Verification items for the finished model (mm, model axes). Face numbers are marked on the shaded views. A direction names the side the tool comes from. Give positions to 0.01 mm unless a question says otherwise; leave off trailing zeros. Loops run counter-clockwise (first coordinate to the right, second up) from the corner with the lowest first, then second, coordinate; pieces in that order, holes last. Notation, with made-up numbers: (50.5, 82.5) -> (69.5, 82.5) arc R17 ccw to (69.5, 110.5) -> close; hole circle Ø11 at (5.5, -5). An arc over 180 degrees is marked (long way). Answer in a Markdown table with one row per item. Add a question column.
Q1. Section check C-C on z = 15.75. Enter the section's corners in (x, y).
Q2. Gauge pin test, flat ends, axial feed: P1, Ø2, axis at x = 29, y = 16, coming from the +Z side; P2, Ø6, axis at y = -17.5, z = 4, coming from the -X side. Record the tip position at first contact, or that the pin passes through.
Q3. Section check A-A on y = -22.5. Enter the section's corners in (x, z), and give its area (3 significant figures).
Q4. Section check D-D on y = -3. Enter the section's corners in (x, z), and give its area (3 significant figures).
Q5. Set-up check for the marked faces 1, 2 and 3: record each of +Z, -Z, +X, -X, +Y, -Y from which the full face is reachable in a straight line by a thin tool's end or side.
Q6. Material ranges on probe 1 along Y at (x, z) = (-17, 12.5); probe 2 along X at (y, z) = (19, 14.5); probe 3 along Y at (x, z) = (-24, 7.75), recorded low to high.
Q7. Release check for a two-part mould opening along X. For the marked faces 4, 5 and 6 record: pulls with the +X half, pulls with the -X half, needs draft (parallel to the pull), parting line crosses it, or undercut.
Q8. Section check B-B on x = 12. Enter the section's corners in (y, z), and give its area (3 significant figures).
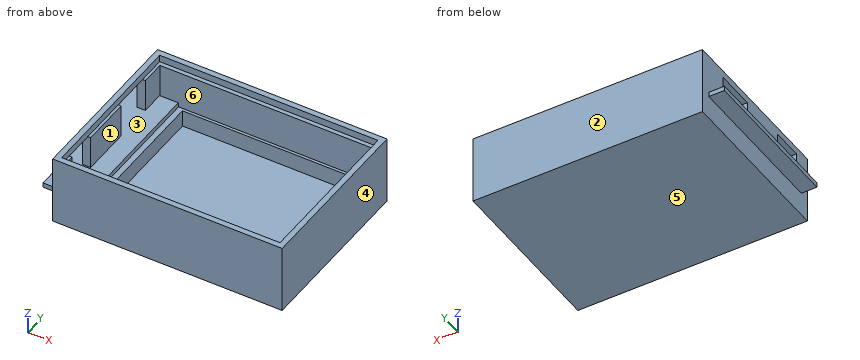
```python
from build123d import *

# Parameters (mm, degrees)
F0_W      = 81.8
F0_H      = 61.16
F1_DEPTH  = 24.5
F2_W      = 77.8
F2_H      = 57.16
F3_DEPTH  = 2.5
F4_W      = 75.8
F4_H      = 54.16
F5_DEPTH  = 13.5
F6_W      = 66.16
F6_H      = 52.16
F7_DEPTH  = 6
F8_W      = 15.217356
F8_H      = 54.009464
F9_DEPTH  = 1.7
F10_W     = 14.16
F10_H     = 11.8
F10_W_2   = 10.9
F11_DEPTH = 4


with BuildPart() as f1:
    # F0 (on Top) → F1 (new body)
    with BuildSketch(Plane.XY):
        Rectangle(F0_W, F0_H)
    extrude(amount=F1_DEPTH)

    # F2 (on face) → F3 (cut)
    with BuildSketch(Plane.XY.offset(24.5)):
        Rectangle(F2_W, F2_H)
    extrude(amount=-F3_DEPTH, mode=Mode.SUBTRACT)

    # F4 (on face) → F5 (cut)
    with BuildSketch(Plane.XY.offset(22)):
        Rectangle(F4_W, F4_H)
    extrude(amount=-F5_DEPTH, mode=Mode.SUBTRACT)

    # F6 (on face) → F7 (cut)
    with BuildSketch(Plane.XY.offset(8.5)):
        with Locations((3.82, 0)):
            Rectangle(F6_W, F6_H)
    extrude(amount=-F7_DEPTH, mode=Mode.SUBTRACT)

    # F8 (on face) → F9 (join)
    with BuildSketch(Plane.XY.offset(8.5)):
        with Locations((-38.868678, -0.085647)):
            Rectangle(F8_W, F8_H)
    extrude(amount=F9_DEPTH)

    # F10 (on face) → F11 (cut)
    with BuildSketch(Plane(origin=(-40.9, 0, 0), x_dir=(0, -1, 0), z_dir=(-1, 0, 0))):
        with Locations((-11.5, 16.1)):
            Rectangle(F10_W, F10_H)
        with Locations((18.77, 16.1)):
            Rectangle(F10_W_2, F10_H)
    extrude(amount=-F11_DEPTH, mode=Mode.SUBTRACT)


solid = f1.part
```
Taken from the geometry:
| question | item | result |
|---|---|---|
| 1 | outline | (-40.9, -30.58) -> (40.9, -30.58) -> (40.9, 30.58) -> (-40.9, 30.58) -> (-40.9, 18.58) -> (-37.9, 18.58) -> (-37.9, 27.08) -> (37.9, 27.08) -> (37.9, -27.08) -> (-37.9, -27.08) -> (-37.9, -24.22) -> (-40.9, -24.22) -> close; (-40.9, -13.32) -> (-37.9, -13.32) -> (-37.9, 4.42) -> (-40.9, 4.42) -> close |
| 2 | P1 | stops at z = 2.5 |
| 2 | P2 | stops at x = -40.9 |
| 3 | outline | (-46.48, 8.5) -> (-40.9, 8.5) -> (-40.9, 0) -> (40.9, 0) -> (40.9, 24.5) -> (38.9, 24.5) -> (38.9, 22) -> (37.9, 22) -> (37.9, 8.5) -> (36.9, 8.5) -> (36.9, 2.5) -> (-29.26, 2.5) -> (-29.26, 8.5) -> (-31.26, 8.5) -> (-31.26, 10.2) -> (-46.48, 10.2) -> close; (-40.9, 22) -> (-38.9, 22) -> (-38.9, 24.5) -> (-40.9, 24.5) -> close |
| 3 | area | 375 mm² |
| 4 | outline | (-46.48, 8.5) -> (-40.9, 8.5) -> (-40.9, 0) -> (40.9, 0) -> (40.9, 24.5) -> (38.9, 24.5) -> (38.9, 22) -> (37.9, 22) -> (37.9, 8.5) -> (36.9, 8.5) -> (36.9, 2.5) -> (-29.26, 2.5) -> (-29.26, 8.5) -> (-31.26, 8.5) -> (-31.26, 10.2) -> (-37.9, 10.2) -> (-37.9, 22) -> (-38.9, 22) -> (-38.9, 24.5) -> (-40.9, 24.5) -> (-40.9, 10.2) -> (-46.48, 10.2) -> close |
| 4 | area | 410 mm² |
| 5 | face 1 | +Z |
| 5 | face 2 | +Z, -Z, +X, -X, +Y |
| 5 | face 3 | none |
| 6 | probe 1 | y = -30.58 to -27.08, 27.08 to 30.58 |
| 6 | probe 2 | x = -40.9 to -37.9, 37.9 to 40.9 |
| 6 | probe 3 | y = -30.58 to -26.08, 26.08 to 30.58 |
| 7 | face 4 | pulls with the +X half |
| 7 | face 5 | needs draft |
| 7 | face 6 | undercut |
| 8 | outline | (-30.58, 0) -> (30.58, 0) -> (30.58, 24.5) -> (28.58, 24.5) -> (28.58, 22) -> (27.08, 22) -> (27.08, 8.5) -> (26.08, 8.5) -> (26.08, 2.5) -> (-26.08, 2.5) -> (-26.08, 8.5) -> (-27.08, 8.5) -> (-27.08, 22) -> (-28.58, 22) -> (-28.58, 24.5) -> (-30.58, 24.5) -> close |
| 8 | area | 311 mm² |
